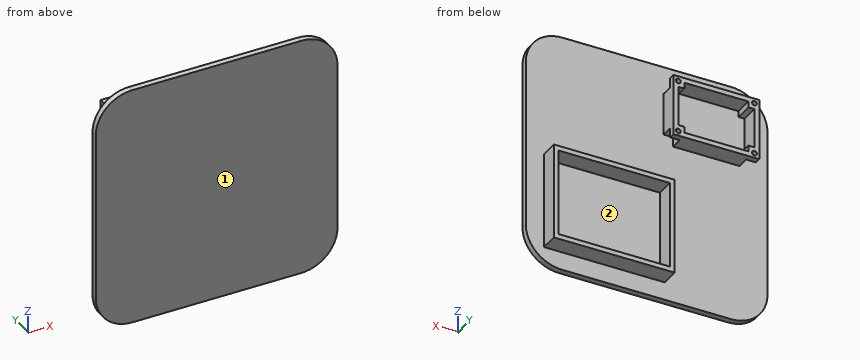
```python
from build123d import *

# Parameters (mm, degrees)
SKETCH1_W            = 200
SKETCH1_H            = 200
BOSS_EXTRUDE1_DEPTH  = 5
SKETCH4_W            = 100
SKETCH4_H            = 80
SKETCH4_W_2          = 92
SKETCH4_H_2          = 72
BOSS_EXTRUDE2_DEPTH  = 15
SKETCH8_W            = 71
SKETCH8_H            = 51
SKETCH8_R            = 2
BOSS_EXTRUDE4_DEPTH  = 15
SKETCH9_W            = 8
SKETCH9_H            = 8
CUT_EXTRUDE11_DEPTH  = 10
LPATTERN1_COUNT      = 2
LPATTERN1_PITCH      = 63
LPATTERN1_COUNT_DIR2 = 2
LPATTERN1_PITCH_DIR2 = 43
FILLET1_R            = 30


with BuildPart() as part:
    # Sketch1 → Boss-Extrude1 (new body)
    with BuildSketch(Plane(origin=(0, 0, 0), x_dir=(1, 0, 0), z_dir=(0, 1, 0))):
        with Locations((100, 100)):
            Rectangle(SKETCH1_W, SKETCH1_H)
    extrude(amount=BOSS_EXTRUDE1_DEPTH)

    # Sketch4 → Boss-Extrude2 (add)
    with BuildSketch(Plane(origin=(0, 5, 0), x_dir=(1, 0, 0), z_dir=(0, 1, 0))):
        with Locations((135, 145)):
            Rectangle(SKETCH4_W, SKETCH4_H)
        with Locations((135, 145)):
            Rectangle(SKETCH4_W_2, SKETCH4_H_2, mode=Mode.SUBTRACT)
    extrude(amount=BOSS_EXTRUDE2_DEPTH)

    # Sketch8 → Boss-Extrude4 (add)
    with BuildSketch(Plane(origin=(0, 5, 0), x_dir=(1, 0, 0), z_dir=(0, 1, 0))):
        with Locations((50.5, 40.5)):
            Rectangle(SKETCH8_W, SKETCH8_H)
        with Locations((19, 62)):
            Circle(SKETCH8_R, mode=Mode.SUBTRACT)
        with Locations((82, 62)):
            Circle(SKETCH8_R, mode=Mode.SUBTRACT)
        with Locations((82, 19)):
            Circle(SKETCH8_R, mode=Mode.SUBTRACT)
        with Locations((19, 19)):
            Circle(SKETCH8_R, mode=Mode.SUBTRACT)
        Polygon((19, 57), (24, 57), (24, 62), (77, 62), (77, 57), (82, 57), (82, 24), (77, 24), (77, 19), (24, 19), (24, 24), (19, 24), align=None, mode=Mode.SUBTRACT)
    extrude(amount=BOSS_EXTRUDE4_DEPTH)

    # Sketch9 → Cut-Extrude11 (cut)
    with BuildSketch(Plane(origin=(0, 5, 0), x_dir=(1, 0, 0), z_dir=(0, 1, 0))):
        with Locations((19, 62)):
            Rectangle(SKETCH9_W, SKETCH9_H)
    cut_extrude11 = extrude(amount=CUT_EXTRUDE11_DEPTH, mode=Mode.SUBTRACT)

    # LPattern1: Cut-Extrude11 2 × 2
    with Locations(*[(i * LPATTERN1_PITCH, 0, j * LPATTERN1_PITCH_DIR2) for i in range(LPATTERN1_COUNT) for j in range(LPATTERN1_COUNT_DIR2) if (i, j) != (0, 0)]):
        add(cut_extrude11, mode=Mode.SUBTRACT)

    # Fillet1
    fillet1_edges = [part.edges().sort_by_distance(p)[0] for p in [
        (0, 2.5, -200),
        (200, 2.5, -200),
        (200, 2.5, 0),
        (0, 2.5, 0),
    ]]
    fillet(fillet1_edges, radius=FILLET1_R)


solid = part.part
```
The model under review builds one solid part; all positions refer to its coordinate system, in mm. Face numbers are marked on the shaded views. Round coordinates to 2 decimals unless told otherwise and drop trailing zeros. Order: outer loops, then holes, each group sorted by start corner. A loop starts at its lowest first (then second) coordinate and runs counter-clockwise, first axis right, second up.
Item 1: For pin 1 (3 mm diameter, centred on x = 155.5, z = -69.5, fed in from +Y); pin 2 (4.5 mm diameter, centred on y = 9, z = -141.5, fed in from +X); pin 3 (2 mm diameter, centred on y = 17.5, z = -105, fed in from -X), all flat-tipped, find the tip position at first contact; note any pin that passes through.
Working result:
pin 1: stops at y = 5
pin 2: stops at x = 185
pin 3: stops at x = 85
Item 2: Add section C-C, the plane z = -77. State the section outline as (x, y) points.
Working result:
outline: (0, 0) - (200, 0) - (200, 5) - (0, 5) - close
Item 3: To check wall thickness, follow probe 1 along X at (y, z) = (8.25, -146.5); probe 2 along X at (y, z) = (16.5, -35); probe 3 along Z at (x, y) = (174, 8). State the ranges of each line that lie inside material, in increasing order.
Working result:
probe 1: x = 85 to 89, 181 to 185
probe 2: x = 15 to 19, 82 to 86
probe 3: z = -185 to -181, -109 to -105
Item 4: Add section A-A, the plane x = 70.5. State the section outline as (y, z) points.
Working result:
outline: (0, -200) - (5, -200) - (5, -66) - (20, -66) - (20, -62) - (5, -62) - (5, -19) - (20, -19) - (20, -15) - (5, -15) - (5, 0) - (0, 0) - close
Item 5: Draft analysis for pull direction Z (two halves, no side actions). For the marked faces 1 and 2, state which applies: released by +Z, released by -Z, zero draft, split by the parting line, or undercut.
Working result:
face 1: zero draft
face 2: undercut
Item 6: Add section B-B, the plane z = -176. State the section outline as (x, y) points, and give its area (3 significant figures).
Working result:
outline: (0.61, 0) - (199.39, 0) - (199.39, 5) - (185, 5) - (185, 20) - (181, 20) - (181, 5) - (89, 5) - (89, 20) - (85, 20) - (85, 5) - (0.61, 5) - close
area: 1,110 mm2
